Source: CAD feature listing. Evaluate the final solid. Frame: model axes, mm. Face numbers are marked on the shaded views. A direction names the side the tool comes from. Give positions to 0.01 mm unless a question says otherwise; leave off trailing zeros. Order: outer loops, then holes, each group sorted by start corner. A loop starts at its lowest first (then second) coordinate and runs counter-clockwise, first axis right, second up.
1) Section A-A, the plane z = 82. Return loops of the section in (x, y).
2) Section C-C, the plane z = -10. Return loops of the section in (x, y).
3) Draft query along Y for the marked faces 1, 2 and 3. Return one class per face: released by +Y, released by -Y, zero draft, split by the parting line, or undercut.
4) Section D-D, the plane y = -136. Return loops of the section in (x, z), plus the area to 3 significant figures.
5) Material intervals for line 1 (Y direction, x = -4, z = 32); line 2 (Z direction, x = -7, y = -258); line 3 (Z direction, x = -7, y = -193), sorted ascending.
6) Access query for the marked faces 4, 5 and 6. Directions: +Z, -Z, +X, -X, +Y, -Y. A direction counts if a zero-diameter tool reaches every point of the face in a straight line with its end or side. Return the directions, or none.
7) Section B-B, the plane y = -258. Return loops of the section in (x, z), plus the area to 3 significant figures.
8) First-contact query: P1, Ø9, axis at y = -258, z = 82, coming from the +X side; P2, Ø10, axis at x = -75.5, z = 34.5, coming from the -Y side; P3, Ø8, axis at y = -233.5, z = 87.5, coming from the -X side; P4, Ø1, axis at x = -79.5, z = 85, coming from the -Y side. Flat tips, straight axial feed; report the tip coordinate or a pass-through.
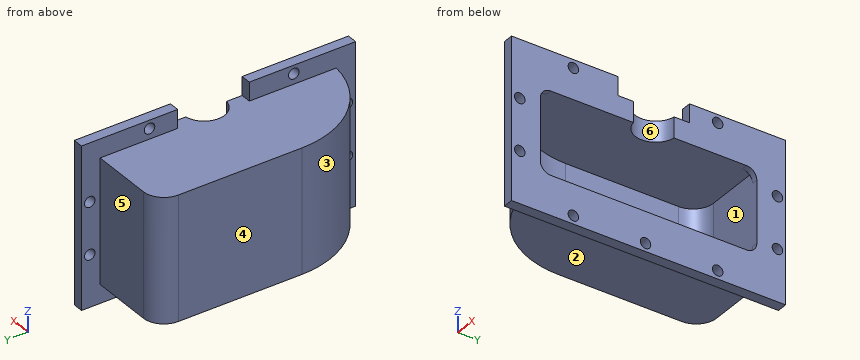
```python
from build123d import *
from build123d.topology import SkipClean

# Parameters (mm, degrees)
BOSS_EXTRUDE2_DEPTH     = 120
CUT_EXTRUDE1_DEPTH      = 10
CUT_EXTRUDE1_DEPTH_BACK = 18
BOSS_EXTRUDE3_DEPTH     = 10
F_1_0MM_DOWEL_HOLE1_D   = 10.2
SKETCH8_W               = 18
SKETCH8_H               = 69.5
CUT_EXTRUDE2_DEPTH      = 10
CUT_EXTRUDE3_START      = -20
CUT_EXTRUDE3_DEPTH      = 20
CUT_EXTRUDE4_DEPTH      = 80
CUT_EXTRUDE5_DEPTH      = 6


with BuildPart() as part:
    # Sketch2 → Boss-Extrude2 (new body)
    with BuildSketch(Plane.XY):
        with BuildLine():
            Line((0, -67.773719933), (0, -28))
            Line((0, -28), (-60, -28))
            ThreePointArc((-60, -28), (-74.142135624, -33.857864376), (-80, -48))
            Line((-80, -48), (-80, -157.773719933))
            ThreePointArc((-80, -157.773719933), (-56.568542495, -214.342262428), (0, -237.773719933))
            Line((0, -237.773719933), (0, -147.773719933))
            Line((0, -147.773719933), (0, -108.226280067))
            Line((0, -108.226280067), (0, -77.773719933))
            Line((0, -77.773719933), (0, -67.773719933))
        make_face()
        with BuildLine():
            Line((0, -28), (0, 0))
            Line((0, 0), (-10, 0))
            Line((-10, 0), (-10, -18))
            Line((-10, -18), (-70, -18))
            ThreePointArc((-70, -18), (-84.142135624, -23.857864376), (-90, -38))
            Line((-90, -38), (-90, -157.773719933))
            ThreePointArc((-90, -157.773719933), (-67.082039325, -217.773719933), (-10, -247.216439033))
            Line((-10, -247.216439033), (-10, -266))
            Line((-10, -266), (0, -266))
            Line((0, -266), (0, -237.773719933))
            ThreePointArc((0, -237.773719933), (-56.568542495, -214.342262428), (-80, -157.773719933))
            Line((-80, -157.773719933), (-80, -48))
            ThreePointArc((-80, -48), (-74.142135624, -33.857864376), (-60, -28))
            Line((-60, -28), (0, -28))
        make_face()
    extrude(amount=BOSS_EXTRUDE2_DEPTH)

    # Sketch3 → Cut-Extrude1 (cut, two sides: drawn at the far end of the back side and taken through both)
    with BuildSketch(Plane.XY.offset(120).offset(-CUT_EXTRUDE1_DEPTH_BACK)):
        with BuildLine():
            Line((0, -147.773719933), (0, -108.226280067))
            ThreePointArc((0, -108.226280067), (-17, -128), (0, -147.773719933))
        make_face()
    extrude(amount=CUT_EXTRUDE1_DEPTH + CUT_EXTRUDE1_DEPTH_BACK, mode=Mode.SUBTRACT)

    # Sketch5 → Boss-Extrude3 (add)
    with BuildSketch(Plane.ZY.offset(10)):
        Polygon((0, -266), (-18, -266), (-18, 0), (138, 0), (138, -266), (120, -266), align=None)
    extrude(amount=-BOSS_EXTRUDE3_DEPTH)

    # Ø1.0mm Dowel Hole1 (through all)
    with Locations(Plane.ZY.offset(10)):
        with Locations((32, -8), (82, -8), (-10, -66), (-10, -136), (-10, -206), (32, -258), (82, -258), (130, -206), (130, -66)):
            Hole(F_1_0MM_DOWEL_HOLE1_D / 2)

    # Sketch8 → Cut-Extrude2 (cut)
    with BuildSketch(Plane.ZY.offset(10)):
        with Locations((129, -128.05)):
            Rectangle(SKETCH8_W, SKETCH8_H)
    extrude(amount=-CUT_EXTRUDE2_DEPTH, mode=Mode.SUBTRACT)

    # Sketch9 → Cut-Extrude3 (cut)
    with SkipClean():  # the faces are left unmerged after this step: merging them gives an invalid solid
        with BuildSketch(Plane.XY.offset(120).offset(CUT_EXTRUDE3_START)):
            with BuildLine():
                Line((0, -147.773719933), (0, -108.226280067))
                ThreePointArc((0, -108.226280067), (-5.320621257, -109.812991947), (-10, -112.801315846))
                Line((-10, -112.801315846), (-10, -143.198684154))
                ThreePointArc((-10, -143.198684154), (-5.320621257, -146.187008053), (0, -147.773719933))
            make_face()
            with BuildLine():
                ThreePointArc((-10, -143.198684154), (-17, -128), (-10, -112.801315846))
                Line((-10, -112.801315846), (-10, -143.198684154))
            make_face()
        extrude(amount=CUT_EXTRUDE3_DEPTH, mode=Mode.SUBTRACT)

    # Sketch12 → Cut-Extrude4 (cut)
    with BuildSketch(Plane(origin=(0, 0, 20), x_dir=(-1, 0, 0), z_dir=(0, 0, -1))):
        with BuildLine():
            Line((60, -28), (6, -28))
            Line((6, -28), (6, -237.548402634))
            ThreePointArc((6, -237.548402634), (58.651513194, -212.179601968), (80, -157.773719933))
            Line((80, -157.773719933), (80, -48))
            ThreePointArc((80, -48), (74.142135624, -33.857864376), (60, -28))
        make_face()
    extrude(amount=-CUT_EXTRUDE4_DEPTH, mode=Mode.SUBTRACT)

    # Sketch10 → Cut-Extrude5 (cut)
    with BuildSketch(Plane(origin=(0, 0, 0), x_dir=(0, 0, -1), z_dir=(1, 0, 0))):
        with BuildLine():
            Line((-30, -238), (-90, -238))
            ThreePointArc((-90, -238), (-97.071067812, -235.071067812), (-100, -228))
            Line((-100, -228), (-100, -38))
            ThreePointArc((-100, -38), (-97.071067812, -30.928932188), (-90, -28))
            Line((-90, -28), (-30, -28))
            ThreePointArc((-30, -28), (-22.928932188, -30.928932188), (-20, -38))
            Line((-20, -38), (-20, -228))
            ThreePointArc((-20, -228), (-22.928932188, -235.071067812), (-30, -238))
        make_face()
    extrude(amount=-CUT_EXTRUDE5_DEPTH, mode=Mode.SUBTRACT)


solid = part.part
```
From the geometry:
1. outline: (-90, -157.77) arc R90 ccw to (-10, -247.22) - (-10, -252.9) - (0, -252.9) - (0, -238) - (-6, -238) - (-6, -237.55) arc R80 cw to (-80, -157.77) - (-80, -48) arc R20 cw to (-60, -28) - (0, -28) - (0, -13.1) - (-10, -13.1) - (-10, -18) - (-70, -18) arc R20 ccw to (-90, -38) - close; (-10, -266) - (0, -266) - (0, -263.1) - (-10, -263.1) - close; (-10, -2.9) - (0, -2.9) - (0, 0) - (-10, 0) - close
2. outline: (-10, -266) - (0, -266) - (0, -211.1) - (-10, -211.1) - close; (-10, -200.9) - (0, -200.9) - (0, -141.1) - (-10, -141.1) - close; (-10, -130.9) - (0, -130.9) - (0, -71.1) - (-10, -71.1) - close; (-10, -60.9) - (0, -60.9) - (0, 0) - (-10, 0) - close
3. face 1: undercut
3. face 2: zero draft
3. face 3: released by -Y
4. outline: (-90, 0) - (-10, 0) - (-10, -4.9) - (0, -4.9) - (0, 20) - (-80, 20) - (-80, 100) - (-15.33, 100) - (-15.33, 120) - (-90, 120) - close; (-10, -18) - (0, -18) - (0, -15.1) - (-10, -15.1) - close
4. area: 4,170 mm2
5. line 1: y = -266 to -263.1, -252.9 to -238, -28 to -13.1, -2.9 to 0
5. line 2: z = -18 to 26.9, 37.1 to 76.9, 87.1 to 138
5. line 3: z = -18 to 20, 100 to 138
6. face 4: +Z, -Z, -X, +Y, -Y
6. face 5: +Z, -Z, -X, +Y
6. face 6: +Z, +X
7. outline: (-10, -18) - (0, -18) - (0, 26.9) - (-10, 26.9) - close; (-10, 37.1) - (0, 37.1) - (0, 76.9) - (-10, 76.9) - close; (-10, 87.1) - (0, 87.1) - (0, 138) - (-10, 138) - close
7. area: 1,360 mm2
8. P1: passes through
8. P2: stops at y = -213.72
8. P3: stops at x = -54.36
8. P4: stops at y = -200.89
